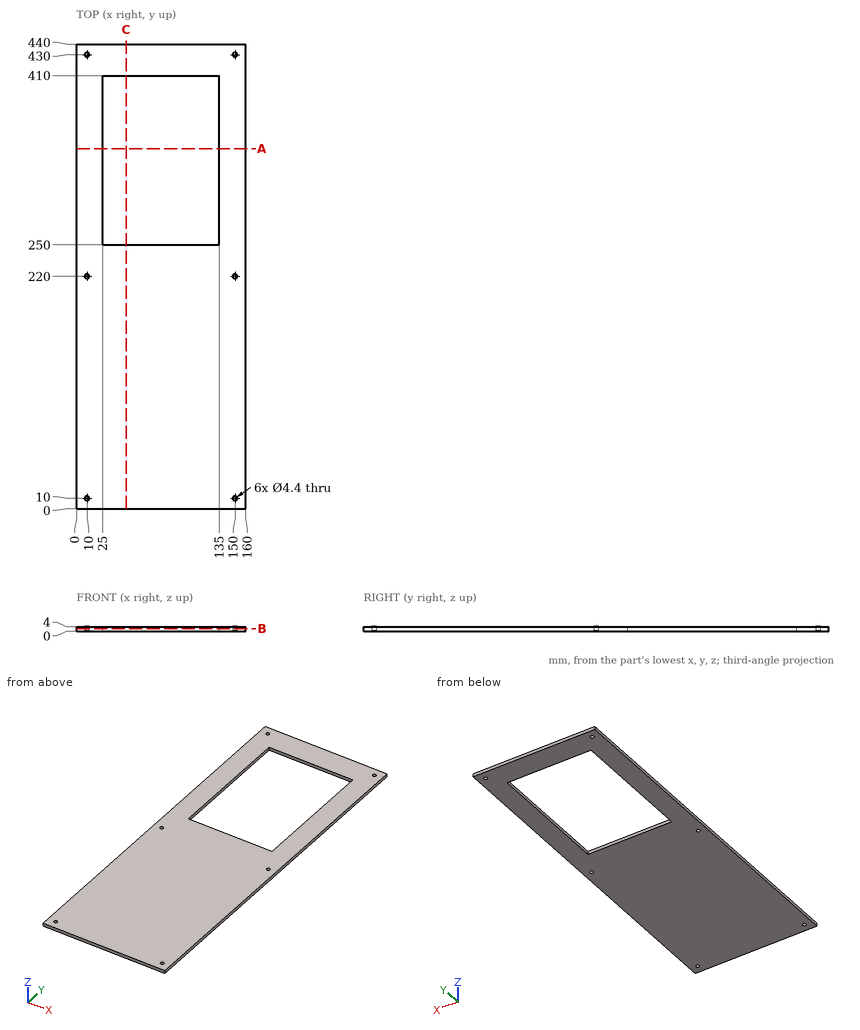
Can you work these out from the drawing? Everything is in mm from the part's minimum corner. Give positions to 0.01 mm unless a question says otherwise; leave off trailing zeros. Write each loop counter-clockwise with the first axis right and the second up, starting at its lowest first coordinate (ties: lowest second). Pieces come first, ordered by that corner, then holes. Notation, with made-up numbers: M -4.5,43.25 L 13.5,43.25 A19 ccw 13.5,54.25 Z; hole C 54.5,17.25 d8. An arc over 180 degrees is marked long. Answer in a Markdown table with one row per item. Add a question column.
Item 1: For pin 1 Ø2 at (x, z) = (34.5, 3) entering from -Y, with a flat end and sliding along its axis, tell me the tip position at first contact or that it passes through.
Item 2: Please list where these lines run through material, in increasing order: L1, parallel to X at y = 220, z = 1.65; L2, parallel to Y at x = 10, z = 2.05; L3, parallel to Y at x = 98, z = 0.75.
Item 3: Imagine slicing it at A-A, the plane y = 341. Write out the boundary of the cut face in (x, z), plus the area to 3 significant figures.
Item 4: Imagine slicing it at B-B, the plane z = 2.35. Write out the boundary of the cut face in (x, y).
Item 5: Imagine slicing it at C-C, the plane x = 47. Write out the boundary of the cut face in (y, z).
Evaluation:
| question | item | result |
|---|---|---|
| 1 | pin 1 | stops at y = 0 |
| 2 | L1 | x = 0 to 7.8, 12.2 to 147.8, 152.2 to 160 |
| 2 | L2 | y = 0 to 7.8, 12.2 to 217.8, 222.2 to 427.8, 432.2 to 440 |
| 2 | L3 | y = 0 to 250, 410 to 440 |
| 3 | outline | M 0,0 L 25,0 L 25,4 L 0,4 Z; M 135,0 L 160,0 L 160,4 L 135,4 Z |
| 3 | area | 200 mm² |
| 4 | outline | M 0,0 L 160,0 L 160,440 L 0,440 Z; hole C 10,10 d4.4; hole C 10,220 d4.4; hole C 10,430 d4.4; hole M 25,250 L 135,250 L 135,410 L 25,410 Z; hole C 150,10 d4.4; hole C 150,220 d4.4; hole C 150,430 d4.4 |
| 5 | outline | M 0,0 L 250,0 L 250,4 L 0,4 Z; M 410,0 L 440,0 L 440,4 L 410,4 Z |
